Autodesk Inventor part; units mm, degrees
ref_plane "YZ Plane" through (0, 0, 0) normal (1, 0, 0) x (0, 1, 0)
ref_plane "XZ Plane" through (0, 0, 0) normal (0, 1, 0) x (-1, 0, 0)
ref_plane "XY Plane" through (0, 0, 0) normal (0, 0, 1) x (1, 0, 0)
sketch "Sketch1" plane through (0, 0, 0) normal (0, 0, 1) x (1, 0, 0)
  line L0 (-114.3, -12.7) -> (114.3, -12.7)
  line L1 (114.3, 12.7) -> (-114.3, 12.7)
  line L2 (-127, -12.7) -> (127, 12.7) construction
  line L3 (127, -12.7) -> (-127, 12.7) construction
  line L4 (-93.6811, -0.2452) -> (-97.6405, -7.1032)
  line L5 (-97.6405, -7.1032) -> (-105.5595, -7.1032)
  line L6 (-105.5595, -7.1032) -> (-109.5189, -0.2452)
  line L7 (-109.5189, -0.2452) -> (-105.5595, 6.6128)
  line L8 (-105.5595, 6.6128) -> (-97.6405, 6.6128)
  line L9 (-97.6405, 6.6128) -> (-93.6811, -0.2452)
  arc A0 (-114.3, 12.7) -> (-114.3, -12.7) centre (-114.3, 0) ccw
  arc A1 (114.3, -12.7) -> (114.3, 12.7) centre (114.3, 0) ccw
  point P0 (0, 0)
  point P1 (-101.6, -0.2452)
  dimension "d0" = 254
  dimension "d1" = 25.4
  dimension "d2" = 13.716
  dimension "d14" = 25.4
extrude "Extrusion4" add sketch "Sketch1" along normal mid plane 6.35
properties part number "armForTurningControlWheel" material "PBT Plastic"
Design review of the part built by this model. Coordinates are the model's own, in mm. A direction names the side the tool comes from. Coordinates: 2 decimals unless noted, no trailing zeros. Loops run counter-clockwise (first coordinate to the right, second up) from the corner with the lowest first, then second, coordinate; pieces in that order, holes last.
Q1. Tool access review of faces 1 (the face through (-107.511, -3.722, -0.044)), 2 (the face through (127, 0, 0)): name each direction out of +Z, -Z, +X, -X, +Y, -Y from which nothing blocks a thin tool from reaching the whole face with its end or side.
Reported:
face 1: +Z, -Z
face 2: +Z, -Z, +X
Q2. To check wall thickness, follow line 1 (X direction, y = -5.75, z = -0.5); line 2 (X direction, y = -6, z = -0.25); line 3 (X direction, y = 8.5, z = 2). State the ranges of each line that lie inside material, in increasing order.
Reported:
line 1: x = -125.62 to -106.34, -96.86 to 125.62
line 2: x = -125.49 to -106.2, -97 to 125.49
line 3: x = -123.74 to 123.74
Q3. The part is to be moulded in two halves that separate along Y. For faces 3 (the face through (-2, 0, 3.175)), 4 (the face through (-102, 6.613, 0)), 5 (the face through (2, 12.7, 0)), 6 (the face through (-95.633, -3.626, -0.044)), say which applies: +Y half, -Y half, draft (parallel to the pull), parting line (faces both ways), or undercut.
Reported:
face 3: draft
face 4: undercut
face 5: +Y half
face 6: undercut
Q4. We need section B-B on z = 0. State the section outline as (x, y) points.
Reported:
outline: (-114.3, -12.7) - (114.3, -12.7) arc R12.7 ccw to (114.3, 12.7) - (-114.3, 12.7) arc R12.7 ccw to start; hole (-109.52, -0.25) - (-105.56, -7.1) - (-97.64, -7.1) - (-93.68, -0.25) - (-97.64, 6.61) - (-105.56, 6.61) - close
Q5. For pin 1 (3 mm diameter, centred on y = 7, z = -1, fed in from -X), flat-tipped, find the tip position at first contact; note if it passes through.
Reported:
pin 1: stops at x = -125.75
Q6. We need section A-A on y = 3.75. State the section outline as (x, z) points (3 decimals).
Reported:
outline: (-126.434, -3.175) - (-107.212, -3.175) - (-107.212, 3.175) - (-126.434, 3.175) - close; (-95.988, -3.175) - (126.434, -3.175) - (126.434, 3.175) - (-95.988, 3.175) - close
